from build123d import *

# Parameters (mm, degrees)
SKETCH1_R           = 1
SKETCH1_R_2         = 1.9
SKETCH1_R_3         = 2.1
SKETCH1_R_4         = 2.4
SKETCH1_R_5         = 1.5
SKETCH1_R_6         = 2.6
BOSS_EXTRUDE1_DEPTH = 2
CHAMFER1_SIZE       = 0.1


with BuildPart() as part:
    # Sketch1 → Boss-Extrude1 (new body)
    with BuildSketch(Plane.XY):
        with BuildLine():
            Line((-30.124585833, 2.496893744), (0, 4))
            Line((0, 4), (20.18611256, 2.493062798))
            ThreePointArc((20.18611256, 2.493062798), (22.5, 0), (20.18611256, -2.493062798))
            Line((20.18611256, -2.493062798), (0, -4))
            Line((0, -4), (-30.124585833, -2.496893744))
            ThreePointArc((-30.124585833, -2.496893744), (-32.5, 0), (-30.124585833, 2.496893744))
        make_face()
        with Locations((-30, 0)):
            Circle(SKETCH1_R, mode=Mode.SUBTRACT)
        with Locations((-23, 0)):
            Circle(SKETCH1_R_2, mode=Mode.SUBTRACT)
        with Locations((-18, 0)):
            Circle(SKETCH1_R_3, mode=Mode.SUBTRACT)
        with Locations((-12.5, 0)):
            Circle(SKETCH1_R_4, mode=Mode.SUBTRACT)
        Circle(SKETCH1_R, mode=Mode.SUBTRACT)
        with Locations((20, 0)):
            Circle(SKETCH1_R_5, mode=Mode.SUBTRACT)
        with Locations((-6.5, 0)):
            Circle(SKETCH1_R_6, mode=Mode.SUBTRACT)
        with Locations((6.5, 0)):
            Circle(SKETCH1_R_6, mode=Mode.SUBTRACT)
        with Locations((12.5, 0)):
            Circle(SKETCH1_R_3, mode=Mode.SUBTRACT)
    extrude(amount=BOSS_EXTRUDE1_DEPTH)

    # Chamfer1
    chamfer1_edges = [part.edges().sort_by_distance(p)[0] for p in [
        (10.09305628, -3.246531399, 2),
        (22.5, 0, 2),
        (-31, 0, 0),
        (-31, 0, 2),
        (-24.9, 0, 0),
        (10.09305628, 3.246531399, 2),
        (-24.9, 0, 2),
        (-20.1, 0, 0),
        (-15.062292916, 3.248446872, 2),
        (-20.1, 0, 2),
        (-14.9, 0, 0),
        (-14.9, 0, 2),
        (-1, 0, 0),
        (-1, 0, 2),
        (18.5, 0, 0),
        (18.5, 0, 2),
        (-9.1, 0, 0),
        (-9.1, 0, 2),
        (10.4, 0, 0),
        (10.4, 0, 2),
        (3.9, 0, 0),
        (3.9, 0, 2),
        (-32.5, 0, 2),
        (-15.062292916, 3.248446872, 0),
        (10.09305628, 3.246531399, 0),
        (22.5, 0, 0),
        (10.09305628, -3.246531399, 0),
        (-15.062292916, -3.248446872, 0),
        (-32.5, 0, 0),
        (-15.062292916, -3.248446872, 2),
    ]]
    chamfer(chamfer1_edges, length=CHAMFER1_SIZE)


solid = part.part
Model file for the job. Use its own axes, mm. Give positions to 0.01 mm unless a question says otherwise; leave off trailing zeros. Loops run counter-clockwise (first coordinate to the right, second up) from the corner with the lowest first, then second, coordinate; pieces in that order, holes last.
Item 1: Mould opens along Y. For faces 1 (the face through (10.234, -3.236, 0.987)), 2 (the face through (-29, 0, 1)), 3 (the face through (22.5, 0.1, 1)), 4 (the face through (8.98, 0.78, 0.99)) say: +Y half, -Y half, draft (parallel to the pull), parting line (faces both ways), or undercut.
Check values:
face 1: -Y half
face 2: undercut
face 3: parting line
face 4: undercut
Item 2: Drop a flat-ended pin along its axis: P1, Ø4, axis at x = 6.5, y = 0, coming from the +Z side. Give the stop position or say it passes through.
Check values:
P1: passes through
Item 3: Slice it at D-D (y = 3.25). Write the cut outline in (x, z).
Check values:
outline: (-15.03, 0.1) - (-13.02, 0) - (8.7, 0) - (10.05, 0.1) - (10.05, 1.9) - (8.7, 2) - (-13.02, 2) - (-15.03, 1.9) - close
Item 4: Slice it at A-A (x = -23). Write the cut outline in (y, z).
Check values:
outline: (-2.85, 0.1) - (-2.75, 0) - (-2, 0) - (-1.9, 0.1) - (-1.9, 1.9) - (-2, 2) - (-2.75, 2) - (-2.85, 1.9) - close; (1.9, 0.1) - (2, 0) - (2.75, 0) - (2.85, 0.1) - (2.85, 1.9) - (2.75, 2) - (2, 2) - (1.9, 1.9) - close
Item 5: Drill centre lines: line 1 along Y through (x, z) = (-30, 1.25); line 2 along Y through (x, z) = (-13, 1.75); line 3 along Y through (x, z) = (-1.5, 0.3). Where is each one in solid material? Low to high.
Check values:
line 1: y = -2.5 to -1, 1 to 2.5
line 2: y = -3.35 to -2.35, 2.35 to 3.35
line 3: y = -3.93 to 3.93
Item 6: Slice it at B-B (z = 1.3). Give the number of separate pieces and of enclosed holes in the cut face, plus the area to 3 significant figures.
Check values:
separate pieces: 1
enclosed holes: 9
area: 232 mm2
